For this review, take the finished solid that the model builds, in its own axes (mm). A direction names the side the tool comes from. Coordinates: 2 decimals unless noted, no trailing zeros. Loops run counter-clockwise (first coordinate to the right, second up) from the corner with the lowest first, then second, coordinate; pieces in that order, holes last. Notation, with made-up numbers: M 41,55 L 96,55 A11 ccw 96,72 Z; hole C 3.5,1 d2. An arc over 180 degrees is marked long. Write item = value, one per line.
from build123d import *

# Parameters (mm, degrees)
SCHIZZO1_W                   = 140
SCHIZZO1_H                   = 55
ESTRUSIONE_ESTRUSIONE1_DEPTH = 4
SCHIZZO2_R                   = 14
SCHIZZO2_R_2                 = 2.75
TAGLIO_ESTRUSIONE1_DEPTH     = 151.469265965
RACCORDO1_R                  = 5
SCHIZZO3_R                   = 6.5
TAGLIO_ESTRUSIONE2_DEPTH     = 151.469265965
TAGLIO_ESTRUSIONE3_DEPTH     = 2


with BuildPart() as part:
    # Schizzo1 → Estrusione-Estrusione1 (new body)
    with BuildSketch(Plane.XY):
        with Locations((70, 27.5)):
            Rectangle(SCHIZZO1_W, SCHIZZO1_H)
    extrude(amount=-ESTRUSIONE_ESTRUSIONE1_DEPTH)

    # Schizzo2 → Taglio-Estrusione1 (cut, through all)
    with BuildSketch(Plane.XY):
        with Locations((27.5, 27.5)):
            Circle(SCHIZZO2_R)
        with Locations((6, 6)):
            Circle(SCHIZZO2_R_2)
        with Locations(Location((49, 6, 0), (0, 0, 180))):
            Circle(SCHIZZO2_R_2)
        with Locations((49, 49)):
            Circle(SCHIZZO2_R_2)
        with Locations(Location((6, 49, 0), (0, 0, 180))):
            Circle(SCHIZZO2_R_2)
    extrude(amount=-TAGLIO_ESTRUSIONE1_DEPTH, mode=Mode.SUBTRACT)

    # Raccordo1
    raccordo1_edges = [part.edges().sort_by_distance(p)[0] for p in [
        (140, 55, -2),
        (140, 0, -2),
    ]]
    fillet(raccordo1_edges, radius=RACCORDO1_R)

    # Schizzo3 → Taglio-Estrusione2 (cut, through all)
    with BuildSketch(Plane(origin=(0, 0, -4), x_dir=(-1, 0, 0), z_dir=(0, 0, -1))):
        with Locations((-108.6, 27.5)):
            Circle(SCHIZZO3_R)
        with BuildLine():
            Line((-134.6, 53.5), (-129.6, 53.5))
            ThreePointArc((-129.6, 53.5), (-127.1, 51), (-129.6, 48.5))
            Line((-129.6, 48.5), (-134.6, 48.5))
            ThreePointArc((-134.6, 48.5), (-137.1, 51), (-134.6, 53.5))
        make_face()
        with BuildLine():
            Line((-82.6, 53.5), (-87.6, 53.5))
            ThreePointArc((-87.6, 53.5), (-90.1, 51), (-87.6, 48.5))
            Line((-87.6, 48.5), (-82.6, 48.5))
            ThreePointArc((-82.6, 48.5), (-80.1, 51), (-82.6, 53.5))
        make_face()
        with BuildLine():
            Line((-134.6, 1.5), (-129.6, 1.5))
            ThreePointArc((-129.6, 1.5), (-127.1, 4), (-129.6, 6.5))
            Line((-129.6, 6.5), (-134.6, 6.5))
            ThreePointArc((-134.6, 6.5), (-137.1, 4), (-134.6, 1.5))
        make_face()
        with BuildLine():
            Line((-82.6, 1.5), (-87.6, 1.5))
            ThreePointArc((-87.6, 1.5), (-90.1, 4), (-87.6, 6.5))
            Line((-87.6, 6.5), (-82.6, 6.5))
            ThreePointArc((-82.6, 6.5), (-80.1, 4), (-82.6, 1.5))
        make_face()
    extrude(amount=-TAGLIO_ESTRUSIONE2_DEPTH, mode=Mode.SUBTRACT)

    # Schizzo4 → Taglio-Estrusione3 (cut)
    with BuildSketch(Plane(origin=(0, 0, -4), x_dir=(-1, 0, 0), z_dir=(0, 0, -1))):
        with BuildLine():
            Line((-88.6, 9), (-128.6, 9))
            ThreePointArc((-128.6, 9), (-132.135533906, 10.464466094), (-133.6, 14))
            Line((-133.6, 14), (-133.6, 41))
            ThreePointArc((-133.6, 41), (-132.135533906, 44.535533906), (-128.6, 46))
            Line((-128.6, 46), (-88.6, 46))
            ThreePointArc((-88.6, 46), (-85.064466094, 44.535533906), (-83.6, 41))
            Line((-83.6, 41), (-83.6, 14))
            ThreePointArc((-83.6, 14), (-85.064466094, 10.464466094), (-88.6, 9))
        make_face()
    extrude(amount=-TAGLIO_ESTRUSIONE3_DEPTH, mode=Mode.SUBTRACT)


solid = part.part
Q1. Draft analysis for pull direction X (two halves, no side actions). For faces 1 (the face through (140, 27, -2)), 2 (the face through (137.1, 50.9, -2)), 3 (the face through (69, 28, 0)), state which applies: +X half, -X half, draft (parallel to the pull), parting line (faces both ways), or undercut.
Solved:
face_1 = +X half
face_2 = undercut
face_3 = draft
Q2. Add section B-B (x = 27.5). Write out the cut boundary in (y, z).
Solved:
outline = M 0,-4 L 13.5,-4 L 13.5,0 L 0,0 Z; M 41.5,-4 L 55,-4 L 55,0 L 41.5,0 Z
Q3. Machinability: for faces 4 (the face through (138, 1, -2)), 5 (the face through (132, 6.5, -2)), 6 (the face through (85.03, 10.5, -3.01)), which of the approach directions +Z, -Z, +X, -X, +Y, -Y give a long, thin tool a straight path to every point of the face, cutting with its end or side? Answer none if there is none.
Solved:
face_4 = +Z, -Z, +X, -Y
face_5 = +Z, -Z
face_6 = -Z
Q4. For pin 1 Ø21 at (x, y) = (108.6, 27.5) entering from -Z; pin 2 Ø5 at (x, y) = (49, 49) entering from -Z, all flat-tipped, find the tip position at first contact; note any pin that passes through.
Solved:
pin_1 = -2
pin_2 = through
Q5. For line 1 along Y through (x, z) = (49, -2.9); line 2 along Y through (x, z) = (134, -2.85); line 3 along Y through (x, z) = (104.5, -2.25), list the stretches that pass through material, from the lowest coordinate up.
Solved:
line_1 = 0 to 3.25, 8.75 to 46.25, 51.75 to 55
line_2 = 0 to 1.5, 6.5 to 48.5, 53.5 to 55
line_3 = 0 to 9, 46 to 55
Q6. Add section A-A (x = 6). Write out the cut boundary in (y, z).
Solved:
outline = M 0,-4 L 3.25,-4 L 3.25,0 L 0,0 Z; M 8.75,-4 L 46.25,-4 L 46.25,0 L 8.75,0 Z; M 51.75,-4 L 55,-4 L 55,0 L 51.75,0 Z
Q7. Add section D-D (y = 19). Write out the cut boundary in (x, z).
Solved:
outline = M 0,-4 L 16.38,-4 L 16.38,0 L 0,0 Z; M 38.62,-4 L 83.6,-4 L 83.6,-2 L 133.6,-2 L 133.6,-4 L 140,-4 L 140,0 L 38.62,0 Z
Q8. Add section C-C (z = -1.2). State how many separate pieces and enclosed holes the cut face has, and give its area (3 significant figures).
Solved:
separate_pieces = 1
enclosed_holes = 10
area = 6,670 mm²
